Read the model definition and answer for the solid it produces. Units are mm, in the model's axes. Face numbers are marked on the shaded views. A direction names the side the tool comes from. Give positions to 0.01 mm unless a question says otherwise; leave off trailing zeros. Loops run counter-clockwise (first coordinate to the right, second up) from the corner with the lowest first, then second, coordinate; pieces in that order, holes last. Notation, with made-up numbers: (32.25, 20) - (66.25, 20) arc R28 ccw to (66.25, 44) - close; hole circle Ø10 at (59, -23). An arc over 180 degrees is marked (long way). Write item = value, one per line.
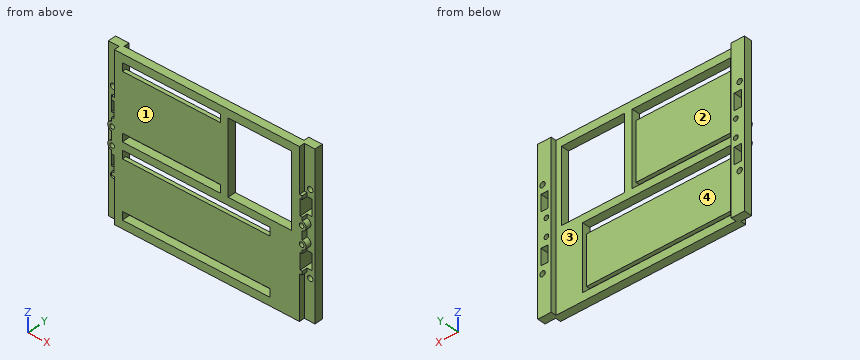
```python
from build123d import *

# Parameters (mm, degrees)
PLATEFRAME_DEPTH          = 150
SKETCH3_R                 = 2.5
HOLESUPPORT_DEPTH         = 13.5
SKETCH4_R                 = 4.15
SKETCH4_R_2               = 2.15
CYLINDRICALSUPPORTS_DEPTH = 12.5
SKETCH8_W                 = 137
SKETCH8_H                 = 60
SKETCH8_W_2               = 91
SKETCH8_H_2               = 68
ITEMLAYOUT_DEPTH          = 4
SKETCH9_W                 = 58.6
SKETCH9_H                 = 68
HOLECUTOUT_DEPTH          = 7.5
SKETCH10_W                = 91
SKETCH10_H                = 7.5
SKETCH10_W_2              = 137
VELCROCUT_DEPTH           = 3.5
SKETCH11_W                = 6.5
SKETCH11_H                = 15
CUTSHELLHOLES_DEPTH       = 12.5
SKETCH12_R                = 2.5
STANDOFFHOLES_DEPTH       = 13.5
SKETCH13_W                = 2.5
SKETCH13_H                = 41
CUTSTANDOFFROOM_DEPTH     = 5


with BuildPart() as part:
    # Sketch2 → PlateFrame (new body)
    with BuildSketch(Plane.XY):
        Polygon((179.1, 12.5), (191.6, 12.5), (191.6, 5), (184.1, 5), (184.1, 0), (7.5, 0), (7.5, 5), (0, 5), (0, 12.5), (12.5, 12.5), (12.5, 7.5), (179.1, 7.5), align=None)
    extrude(amount=PLATEFRAME_DEPTH)

    # Sketch3 → HoleSupport (cut, through all)
    with BuildSketch(Plane(origin=(0, 12.5, 0), x_dir=(1, 0, 0), z_dir=(0, 1, 0))):
        with Locations((8.05, -66.85)):
            Circle(SKETCH3_R)
        with Locations((8.05, -83.15)):
            Circle(SKETCH3_R)
        with Locations((183.55, -66.85)):
            Circle(SKETCH3_R)
        with Locations((183.55, -83.15)):
            Circle(SKETCH3_R)
    extrude(amount=-HOLESUPPORT_DEPTH, mode=Mode.SUBTRACT)

    # Sketch4 → CylindricalSupports (add)
    with BuildSketch(Plane(origin=(0, 12.5, 0), x_dir=(1, 0, 0), z_dir=(0, 1, 0))):
        with Locations((183.55, -66.85)):
            Circle(SKETCH4_R)
        with Locations((183.55, -66.85)):
            Circle(SKETCH4_R_2, mode=Mode.SUBTRACT)
        with Locations((183.55, -83.15)):
            Circle(SKETCH4_R)
        with Locations((183.55, -83.15)):
            Circle(SKETCH4_R_2, mode=Mode.SUBTRACT)
        with Locations((8.05, -66.85)):
            Circle(SKETCH4_R)
        with Locations((8.05, -66.85)):
            Circle(SKETCH4_R_2, mode=Mode.SUBTRACT)
        with Locations((8.05, -83.15)):
            Circle(SKETCH4_R)
        with Locations((8.05, -83.15)):
            Circle(SKETCH4_R_2, mode=Mode.SUBTRACT)
    extrude(amount=-CYLINDRICALSUPPORTS_DEPTH)

    # Sketch8 → ItemLayout (cut)
    with BuildSketch(Plane(origin=(0, 7.5, 0), x_dir=(1, 0, 0), z_dir=(0, 1, 0))):
        with Locations((86, -37.5)):
            Rectangle(SKETCH8_W, SKETCH8_H)
        with Locations((63, -108.5)):
            Rectangle(SKETCH8_W_2, SKETCH8_H_2)
    extrude(amount=-ITEMLAYOUT_DEPTH, mode=Mode.SUBTRACT)

    # Sketch9 → HoleCutout (cut)
    with BuildSketch(Plane(origin=(0, 7.5, 0), x_dir=(1, 0, 0), z_dir=(0, 1, 0))):
        with Locations((144.8, -108.5)):
            Rectangle(SKETCH9_W, SKETCH9_H)
    extrude(amount=-HOLECUTOUT_DEPTH, mode=Mode.SUBTRACT)

    # Sketch10 → VelcroCut (cut)
    with BuildSketch(Plane(origin=(0, 3.5, 0), x_dir=(1, 0, 0), z_dir=(0, 1, 0))):
        with Locations((63, -78.25)):
            Rectangle(SKETCH10_W, SKETCH10_H)
        with Locations((63, -138.75)):
            Rectangle(SKETCH10_W, SKETCH10_H)
        with Locations((86, -11.25)):
            Rectangle(SKETCH10_W_2, SKETCH10_H)
        with Locations((86, -63.75)):
            Rectangle(SKETCH10_W_2, SKETCH10_H)
    extrude(amount=-VELCROCUT_DEPTH, mode=Mode.SUBTRACT)

    # Sketch11 → CutShellHoles (cut)
    with BuildSketch(Plane(origin=(0, 12.5, 0), x_dir=(1, 0, 0), z_dir=(0, 1, 0))):
        with Locations((6.25, -51.85)):
            Rectangle(SKETCH11_W, SKETCH11_H)
        with Locations((185.35, -51.85)):
            Rectangle(SKETCH11_W, SKETCH11_H)
        with Locations((185.35, -98.15)):
            Rectangle(SKETCH11_W, SKETCH11_H)
        with Locations((6.25, -98.15)):
            Rectangle(SKETCH11_W, SKETCH11_H)
    extrude(amount=-CUTSHELLHOLES_DEPTH, mode=Mode.SUBTRACT)

    # Sketch12 → StandoffHoles (cut, through all)
    with BuildSketch(Plane(origin=(0, 12.5, 0), x_dir=(1, 0, 0), z_dir=(0, 1, 0))):
        with Locations((4.5, -36.85)):
            Circle(SKETCH12_R)
        with Locations((4.5, -113.15)):
            Circle(SKETCH12_R)
        with Locations((187.1, -36.85)):
            Circle(SKETCH12_R)
        with Locations((187.1, -113.15)):
            Circle(SKETCH12_R)
    extrude(amount=-STANDOFFHOLES_DEPTH, mode=Mode.SUBTRACT)

    # Sketch13 → CutStandoffRoom (cut)
    with BuildSketch(Plane.XZ):
        with Locations((8.75, 20.5)):
            Rectangle(SKETCH13_W, SKETCH13_H)
        with Locations((8.75, 129.5)):
            Rectangle(SKETCH13_W, SKETCH13_H)
        with Locations((182.85, 129.5)):
            Rectangle(SKETCH13_W, SKETCH13_H)
        with Locations((182.85, 20.5)):
            Rectangle(SKETCH13_W, SKETCH13_H)
    extrude(amount=-CUTSTANDOFFROOM_DEPTH, mode=Mode.SUBTRACT)


solid = part.part
```
1) A cutting plane is placed at C-C on x = 121. Determine the outline of the cut face in (y, z).
Output:
outline = (0, 0) - (7.5, 0) - (7.5, 7.5) - (0, 7.5) - close; (0, 15) - (3.5, 15) - (3.5, 60) - (0, 60) - close; (0, 67.5) - (7.5, 67.5) - (7.5, 74.5) - (0, 74.5) - close; (0, 142.5) - (7.5, 142.5) - (7.5, 150) - (0, 150) - close
2) A cutting plane is placed at B-B on x = 21. Determine the outline of the cut face in (y, z), then the cut area to 3 significant figures.
Output:
outline = (0, 0) - (7.5, 0) - (7.5, 7.5) - (0, 7.5) - close; (0, 15) - (3.5, 15) - (3.5, 60) - (0, 60) - close; (0, 67.5) - (7.5, 67.5) - (7.5, 74.5) - (0, 74.5) - close; (0, 82) - (3.5, 82) - (3.5, 135) - (0, 135) - close; (0, 142.5) - (7.5, 142.5) - (7.5, 150) - (0, 150) - close
area = 508 mm²
3) Find the intervals of material crossed by probe 1 along Z at (x, y) = (4.5, 7); probe 2 along X at (y, z) = (11, 66.5); probe 3 along Z at (x, y) = (45, 1), in increasing order.
Output:
probe_1 = 0 to 34.35, 39.35 to 44.35, 59.35 to 90.65, 105.65 to 110.65, 115.65 to 150
probe_2 = 0 to 5.93, 10.17 to 12.5, 179.1 to 181.43, 185.67 to 191.6
probe_3 = 0 to 7.5, 15 to 60, 67.5 to 74.5, 82 to 135, 142.5 to 150
4) A cutting plane is placed at A-A on z = 126. Determine the outline of the cut face in (x, y), then the cut area to 4 significant figures.
Output:
outline = (0, 5) - (10, 5) - (10, 0) - (115.5, 0) - (115.5, 7.5) - (108.5, 7.5) - (108.5, 3.5) - (17.5, 3.5) - (17.5, 7.5) - (12.5, 7.5) - (12.5, 12.5) - (0, 12.5) - close; (174.1, 0) - (181.6, 0) - (181.6, 5) - (191.6, 5) - (191.6, 12.5) - (179.1, 12.5) - (179.1, 7.5) - (174.1, 7.5) - close
area = 658.5 mm²
5) A tool of negligible diameter and unlimited length cuts with its end or side. For the marked faces 3 and 4, from which of +Z, -Z, +X, -X, +Y, -Y can it reach the whole face along a straight path? Write none if from no direction.
Output:
face_3 = +Z, -Z, +Y
face_4 = +Y
6) Each of these flat-tipped pins is pushed along its axis until it touches: P1, Ø4, axis at x = 83.5, z = 70, coming from the -Y side; P2, Ø1.5, axis at y = 3, z = 14.5, coming from the -X side; P3, Ø2.5, axis at y = 2.5, z = 88, coming from the +X side; P4, Ø1.7, axis at y = 2.5, z = 61.5, coming from the +X side. Where does it stop, or does it pass through?
Output:
P1 = 0
P2 = 10
P3 = 185.61
P4 = 184.1
7) The mould has two halves that part along X. Classify the marked faces 1 and 2: pulls with the +X half, pulls with the -X half, needs draft (parallel to the pull), parting line crosses it, or undercut.
Output:
face_1 = needs draft
face_2 = undercut
